The model under review builds one solid part; all positions refer to its coordinate system, in mm. Round coordinates to 2 decimals unless told otherwise and drop trailing zeros. Order: outer loops, then holes, each group sorted by start corner. A loop starts at its lowest first (then second) coordinate and runs counter-clockwise, first axis right, second up. Notation, with made-up numbers: (35.25, 70.25) - (78.25, 70.25) arc R16 cw to (78.25, 80.25) - close; hole circle Ø5 at (82.25, 37.25). An arc over 180 degrees is marked (long way). One line per question, with ' | ' between items. Start each with the question number.
Item 1: For L1, parallel to X at y = 18.5, z = 24.5; L2, parallel to X at y = 11, z = 26.5; L3, parallel to Y at x = -28.5, z = 46.5, list the stretches that pass through material, from the lowest coordinate up. Write a range as [from, to].
Item 2: Add section A-A on x = -101. State the section outline as (y, z) points.
Item 3: Add section B-B on y = 19. State the section outline as (x, z) points, and give its area (3 significant figures).
Item 4: Draft analysis for pull direction Y (two halves, no side actions). For faces 1 (the face through (-44.76, 64.549, 48.224)), 2 (the face through (-45, -45.434, 23)), 3 (the face through (46.273, 10, 23)), 4 (the face through (-100.153, 10.054, 25.044)), state which applies: +Y half, -Y half, draft (parallel to the pull), parting line (faces both ways), or undercut.
Item 5: Insertion check: pin 1 Ø14.5 at (x, y) = (-101.53, 16.25) entering from -Z. The pin has a flat end and moves straight along its axis. Give the tip position at first contact, or say it passes through.
from build123d import *

# Parameters (mm, degrees)
F0_W     = 179.552953
F0_H     = 112.487468
F1_DEPTH = 50.8
F3_D     = 12.7
F4_SIZE  = 5.08
F5_SIZE  = 5.08


with BuildPart() as f1:
    # F0 (on Top) → F1 (new body)
    with BuildSketch(Plane.XY):
        with Locations((-43.503502, 10.809673)):
            Rectangle(F0_W, F0_H)
    extrude(amount=F1_DEPTH)

    # F3 (through all)
    with Locations(Plane.XY.offset(50.8)):
        with Locations((-101.529979, 16.253407)):
            Hole(F3_D / 2)

    # F4
    f4_edges = [f1.edges().sort_by_distance(p)[0] for p in [
        (-43.503502, -45.434061, 50.8),
    ]]
    chamfer(f4_edges, length=F4_SIZE)

    # F5
    f5_edges = [f1.edges().sort_by_distance(p)[0] for p in [
        (46.272974, 13.349673, 50.8),
        (-43.503502, 67.053407, 50.8),
        (-133.279979, 13.349673, 50.8),
    ]]
    chamfer(f5_edges, length=F5_SIZE)


solid = f1.part
Determined:
1) L1: [-133.28, -107.47], [-95.59, 46.27] | L2: [-133.28, -105.1], [-97.96, 46.27] | L3: [-44.65, 66.27]
2) outline: (-45.43, 0) - (9.93, 0) - (9.93, 50.8) - (-40.35, 50.8) - (-45.43, 45.72) - close; (22.58, 0) - (67.05, 0) - (67.05, 45.72) - (61.97, 50.8) - (22.58, 50.8) - close
3) outline: (-133.28, 0) - (-107.26, 0) - (-107.26, 50.8) - (-128.2, 50.8) - (-133.28, 45.72) - close; (-95.8, 0) - (46.27, 0) - (46.27, 45.72) - (41.19, 50.8) - (-95.8, 50.8) - close | area: 8,510 mm2
4) face 1: +Y half | face 2: -Y half | face 3: draft | face 4: undercut
5) pin 1: z = 0
